Autodesk Inventor part; units mm, degrees
ref_plane "YZ Plane" through (0, 0, 0) normal (1, 0, 0) x (0, 1, 0)
ref_plane "XZ Plane" through (0, 0, 0) normal (0, 1, 0) x (-1, 0, 0)
ref_plane "XY Plane" through (0, 0, 0) normal (0, 0, 1) x (1, 0, 0)
sketch "スケッチ1" plane through (0, 0, 0) normal (1, 0, 0) x (0, 1, 0)
  line L0 (-115.2146, 152.1685) -> (124.7854, 152.1685)
  line L1 (124.7854, 152.1685) -> (114.7854, 152.1685)
  line L2 (114.7854, 152.1685) -> (114.7854, -77.8315)
  line L3 (114.7854, -77.8315) -> (124.7854, -77.8315)
  line L4 (124.7854, -77.8315) -> (124.7854, 152.1685)
  line L5 (-115.2146, 152.1685) -> (-105.2146, 152.1685)
  line L6 (-105.2146, 152.1685) -> (-105.2146, -77.8315)
  line L7 (-105.2146, -77.8315) -> (-115.2146, -77.8315)
  line L8 (-115.2146, -77.8315) -> (-115.2146, 152.1685)
  line L9 (124.7854, 152.1685) -> (124.7854, 162.1685)
  line L10 (-115.2146, 162.1685) -> (124.7854, 162.1685)
  line L11 (4.7854, 162.1685) -> (4.7854, -110.7311)
  line L12 (124.7854, 127.1685) -> (114.7854, 127.1685)
  line L13 (99.7854, 152.1685) -> (99.7854, 162.1685)
  circle A0 centre (119.7854, 137.1685) radius 1.5
  circle A1 centre (119.7854, 147.1685) radius 1.5
  circle A2 centre (119.7854, 157.1685) radius 1.5
  circle A3 centre (109.7854, 157.1685) radius 1.5
  line L14 (114.7854, 152.1685) -> (99.7854, 152.1685)
  line L15 (124.7854, 152.1685) -> (124.7854, 162.1685)
  line L16 (124.7854, 162.1685) -> (99.7854, 162.1685)
  point P0 (0, 0)
  point P1 (4.7854, -147.8315)
  point P2 (-110.2146, 157.1685)
  point P3 (-100.2146, 157.1685)
  point P4 (-110.2146, 147.1685)
  point P5 (-110.2146, 137.1685)
  dimension "d0" = 10
  dimension "d1" = 230
  dimension "d2" = 10
  dimension "d3" = 230
  dimension "d4" = 5
  dimension "d5" = 10
  dimension "d6" = 5
  dimension "d7" = 5
  dimension "d8" = 5
  dimension "d9" = 10
  dimension "d10" = 5
  dimension "d11" = 5
  dimension "d12" = 10
  dimension "d13" = 10
  dimension "d14" = 3
  dimension "d15" = 3
  dimension "d16" = 3
  dimension "d17" = 3
extrude "押し出し1" add sketch "スケッチ1" against normal blind 3 contours L13 L10 L9 L0 | L0 L4 L12 L2
fillet "フィレット1" radius 2 6 edges at (-1.5, 124.7854, 162.1685) (-1.5, 124.7854, 127.1685) (-1.5, 114.7854, 127.1685) (-1.5, 114.7854, 152.1685) (-1.5, 99.7854, 152.1685) (-1.5, 99.7854, 162.1685)
sketch "スケッチ3" plane through (0, 0, 0) normal (1, 0, 0) x (0, 0, -1)
  circle A0 centre (-157.1685, 119.7854) radius 1.5
  circle A1 centre (-157.1685, 109.7854) radius 1.5
  circle A2 centre (-147.1685, 119.7854) radius 1.5
  circle A3 centre (-137.1685, 119.7854) radius 1.5
  arc A4 (-162.1685, 101.7854) -> (-160.1685, 99.7854) centre (-160.1685, 101.7854) ccw
  line L0 (-160.1685, 99.7854) -> (-154.1685, 99.7854)
  arc A5 (-154.1685, 99.7854) -> (-152.1685, 101.7854) centre (-154.1685, 101.7854) ccw
  line L1 (-152.1685, 101.7854) -> (-152.1685, 112.7854)
  arc A6 (-150.1685, 114.7854) -> (-152.1685, 112.7854) centre (-150.1685, 112.7854) ccw
  line L2 (-150.1685, 114.7854) -> (-129.1685, 114.7854)
  arc A7 (-129.1685, 114.7854) -> (-127.1685, 116.7854) centre (-129.1685, 116.7854) ccw
  line L3 (-127.1685, 116.7854) -> (-127.1685, 122.7854)
  arc A8 (-127.1685, 122.7854) -> (-129.1685, 124.7854) centre (-129.1685, 122.7854) ccw
  line L4 (-129.1685, 124.7854) -> (-160.1685, 124.7854)
  arc A9 (-160.1685, 124.7854) -> (-162.1685, 122.7854) centre (-160.1685, 122.7854) ccw
  line L5 (-162.1685, 122.7854) -> (-162.1685, 101.7854)
  point P0 (0, 0)
properties part number "belt_liner_v1_MDF_F_1" material "MDF 中密度繊維ボード"
Part model, mm, in its own coordinate system. A direction names the side the tool comes from. Round coordinates to 2 decimals unless told otherwise and drop trailing zeros. Loops run counter-clockwise (first coordinate to the right, second up) from the corner with the lowest first, then second, coordinate; pieces in that order, holes last.
Item 1: Cut at B-B, the plane z = 141.5. Give the cut face in (x, y), then the cut area to 3 significant figures.
Item 2: 3-axis set-ups, long thin cutter, end or side, ignore diameter. For faces 4 (the face through (-1, 114.785, 140)), 5 (the face through (-1.48, 120.48, 135.84)): which of +Z, -Z, +X, -X, +Y, -Y reach the whole face in a straight line?
Item 3: Drop flat-ended pins along their axis: P1, Ø5, axis at y = 119.79, z = 157.17, coming from the -X side; P2, Ø1.5, axis at x = -1.5, z = 139.5, coming from the -Y side; P3, Ø2.5, axis at y = 109.79, z = 157.17, coming from the -X side. Give the stop position or say it passes through.
Item 4: Drill centre lines: line 1 (Z direction, x = -1.6, y = 119.75); line 2 (Y direction, x = -0.9, z = 156); line 3 (Z direction, x = -1.7, y = 109.75). Where is each one in solid material? Low to high.
Item 5: Mould opens along Z. For faces 1 (the face through (-1, 120, 127.168)), 2 (the face through (-1.479, 119.46, 145.704)), 3 (the face through (-1, 99.785, 157)) say: +Z half, -Z half, draft (parallel to the pull), parting line (faces both ways), or undercut.
Item 6: Cut at A-A, the plane y = 120.25. Give the cut face in (x, z).
Item 7: Cut at C-C, the plane x = -1.05. Give the cut face in (y, z), then the cut area to 3 significant figures.
Item 8: Cut at D-D, the plane y = 107.5. Give the cut face in (x, z).
A:
1. outline: (-3, 114.79) - (0, 114.79) - (0, 124.79) - (-3, 124.79) - close
1. area: 30.0 mm2
2. face 4: -Z, +X, -X, -Y
2. face 5: +X, -X
3. P1: stops at x = -3
3. P2: stops at y = 114.79
3. P3: passes through
4. line 1: z = 127.17 to 135.67, 138.67 to 145.67, 148.67 to 155.67, 158.67 to 162.17
4. line 2: y = 99.79 to 108.84, 110.73 to 118.84, 120.73 to 124.79
4. line 3: z = 152.17 to 155.67, 158.67 to 162.17
5. face 1: -Z half
5. face 2: undercut
5. face 3: draft
6. outline: (-3, 127.17) - (0, 127.17) - (0, 135.74) - (-3, 135.74) - close; (-3, 138.59) - (0, 138.59) - (0, 145.74) - (-3, 145.74) - close; (-3, 148.59) - (0, 148.59) - (0, 155.74) - (-3, 155.74) - close; (-3, 158.59) - (0, 158.59) - (0, 162.17) - (-3, 162.17) - close
7. outline: (99.79, 154.17) arc R2 ccw to (101.79, 152.17) - (112.79, 152.17) arc R2 cw to (114.79, 150.17) - (114.79, 129.17) arc R2 ccw to (116.79, 127.17) - (122.79, 127.17) arc R2 ccw to (124.79, 129.17) - (124.79, 160.17) arc R2 ccw to (122.79, 162.17) - (101.79, 162.17) arc R2 ccw to (99.79, 160.17) - close; hole circle Ø3 at (109.79, 157.17); hole circle Ø3 at (119.79, 137.17); hole circle Ø3 at (119.79, 147.17); hole circle Ø3 at (119.79, 157.17)
7. area: 468 mm2
8. outline: (-3, 152.17) - (0, 152.17) - (0, 162.17) - (-3, 162.17) - close
